```python
from build123d import *

# Parameters (mm, degrees)
SKETCH2_W           = 42
SKETCH2_H           = 80
BOSS_EXTRUDE1_DEPTH = 2
SKETCH5_W           = 31.9
SKETCH5_H           = 70.25
BOSS_EXTRUDE2_DEPTH = 0.5
FILLET1_R           = 3.95
SKETCH7_R           = 11
CUT_EXTRUDE1_DEPTH  = 46.24654683
SKETCH8_R           = 1.6
CUT_EXTRUDE2_DEPTH  = 46.24654683


with BuildPart() as part:
    # Sketch2 → Boss-Extrude1 (new body)
    with BuildSketch(Plane.XY):
        Rectangle(SKETCH2_W, SKETCH2_H)
    extrude(amount=BOSS_EXTRUDE1_DEPTH)

    # Sketch5 → Boss-Extrude2 (add)
    with BuildSketch(Plane.XY.offset(2)):
        Rectangle(SKETCH5_W, SKETCH5_H)
    extrude(amount=BOSS_EXTRUDE2_DEPTH)

    # Fillet1
    fillet1_edges = [part.edges().sort_by_distance(p)[0] for p in [
        (15.95, -35.125, 2.25),
        (15.95, 35.125, 2.25),
        (-15.95, 35.125, 2.25),
        (-15.95, -35.125, 2.25),
    ]]
    fillet(fillet1_edges, radius=FILLET1_R)

    # Sketch7 → Cut-Extrude1 (cut, through all)
    with BuildSketch(Plane.XY.offset(2.5)):
        with Locations((0, 23.875)):
            Circle(SKETCH7_R)
    extrude(amount=-CUT_EXTRUDE1_DEPTH, mode=Mode.SUBTRACT)

    # Sketch8 → Cut-Extrude2 (cut, through all)
    with BuildSketch(Plane(origin=(0, 0, 0), x_dir=(-1, 0, 0), z_dir=(0, 0, -1))):
        with Locations((18, 37)):
            Circle(SKETCH8_R)
        with Locations((-18, 37)):
            Circle(SKETCH8_R)
        with Locations((-18, -37)):
            Circle(SKETCH8_R)
        with Locations((18, -37)):
            Circle(SKETCH8_R)
    extrude(amount=-CUT_EXTRUDE2_DEPTH, mode=Mode.SUBTRACT)


solid = part.part
```
Could you check a few things on this model? Use its own coordinates, in mm. A direction names the side the tool comes from. Coordinates: 2 decimals unless noted, no trailing zeros. Loops run counter-clockwise (first coordinate to the right, second up) from the corner with the lowest first, then second, coordinate; pieces in that order, holes last. Notation, with made-up numbers: M -14.75,-11.75 L 6.25,-11.75 A20 ccw 6.25,14.25 Z; hole C 88.5,65.5 d8. An arc over 180 degrees is marked long. Put each result on its own line as item: value. Start each with the question number.
(1) Suppose I cut it at D-D on y = 3. Please give me the cut outline in (x, z).
(2) Suppose I cut it at C-C on x = 0. Please give me the cut outline in (y, z) (3 decimals).
(3) Suppose I cut it at B-B on x = -18. Please give me the cut outline in (y, z).
(4) Thinking about a two-plate mould opening in Y: for faces 5 (the face through (-14.76, 34, 2.25)), 6 (the face through (-2.385, 13.137, 1.268)), 7 (the face through (0, 1, 0)), which applies, pulls with the +Y half, pulls with the -Y half, needs draft (parallel to the pull), parting line crosses it, or undercut?
(5) I need wall thicknesses on line 1 (Y direction, x = -18, z = 1.3); line 2 (Y direction, x = 0, z = 1.1) (3 decimals); line 3 (X direction, y = 23.5, z = 0.35). Which ranges of each line are inside material? Lowest first, please. Write a range as from..to.
(6) Suppose I cut it at A-A on y = 37. Please give me the cut outline in (x, z).
(7) For faces 1 (the face through (14.76, -34, 2.25)), 2 (the face through (14.82, 33.94, 2.25)), 3 (the face through (-17, 0, 2)), 4 (the face through (-14.76, -34, 2.25)), which set-ups out of +Z, -Z, +X, -X, +Y, -Y let a thin tool reach every point of the face, with its end or its side?
(8) Will this pin go through, and if not, where does the flat tip stop? P1, Ø4, axis at x = 18, y = 37, coming from the +Z side.
Solutions:
1. outline: M -21,0 L 21,0 L 21,2 L 15.95,2 L 15.95,2.5 L -15.95,2.5 L -15.95,2 L -21,2 Z
2. outline: M -40,0 L 12.875,0 L 12.875,2.5 L -35.125,2.5 L -35.125,2 L -40,2 Z; M 34.875,0 L 40,0 L 40,2 L 35.125,2 L 35.125,2.5 L 34.875,2.5 Z
3. outline: M -40,0 L -38.6,0 L -38.6,2 L -40,2 Z; M -35.4,0 L 35.4,0 L 35.4,2 L -35.4,2 Z; M 38.6,0 L 40,0 L 40,2 L 38.6,2 Z
4. face 5: pulls with the +Y half
4. face 6: undercut
4. face 7: needs draft
5. line 1: y = -40..-38.6, -35.4..35.4, 38.6..40
5. line 2: y = -40..12.875, 34.875..40
5. line 3: x = -21..-10.99, 10.99..21
6. outline: M -21,0 L -19.6,0 L -19.6,2 L -21,2 Z; M -16.4,0 L 16.4,0 L 16.4,2 L -16.4,2 Z; M 19.6,0 L 21,0 L 21,2 L 19.6,2 Z
7. face 1: +Z, +X, -Y
7. face 2: +Z, +X, +Y
7. face 3: +Z
7. face 4: +Z, -X, -Y
8. P1: stops at z = 2
